The drawing under review shows one solid part. Ordinate dimensions are in mm from its lowest x, y, z. A direction names the side the tool comes from. Coordinates: 2 decimals unless noted, no trailing zeros. Loops run counter-clockwise (first coordinate to the right, second up) from the corner with the lowest first, then second, coordinate; pieces in that order, holes last.
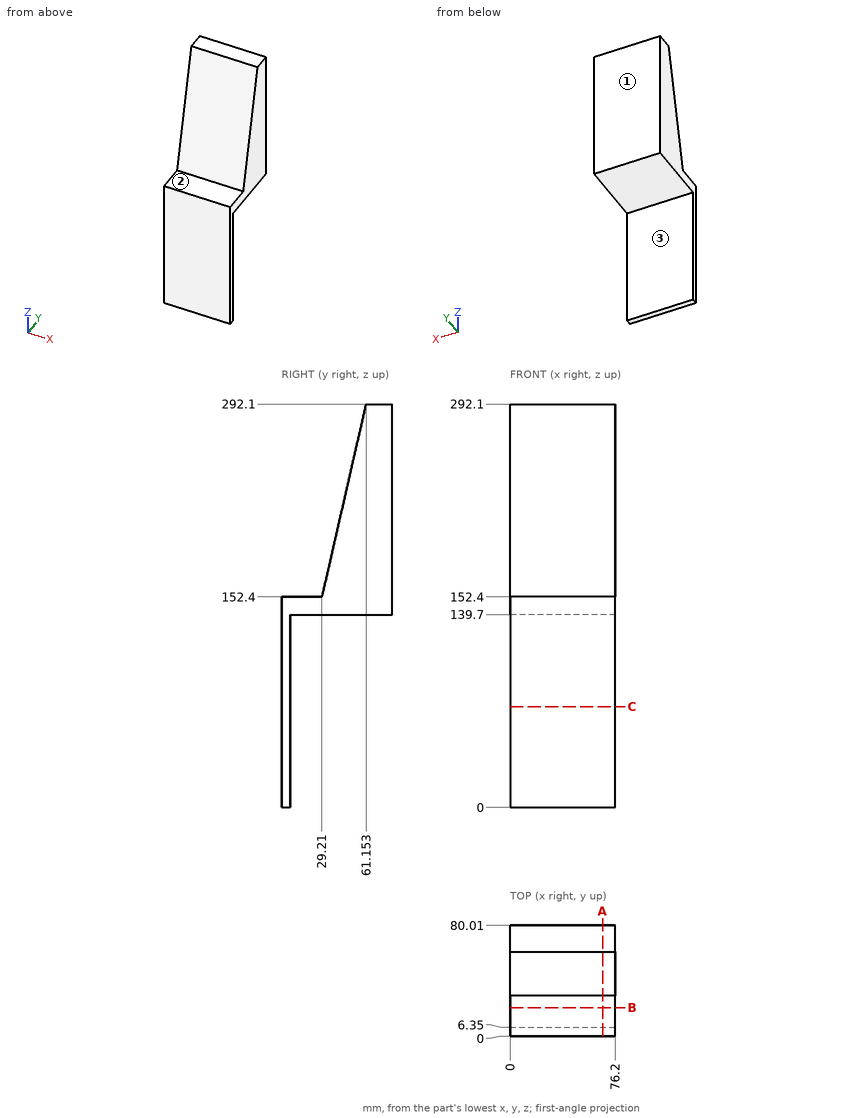
Q1. Take a section at C-C, the plane z = 73. Write out the cut boundary in (x, y).
Q2. Take a section at B-B, the plane y = 20.5. Write out the cut boundary in (x, z).
Q3. Take a section at A-A, the plane x = 67. Write out the cut boundary in (y, z).
Q4. For line 1 (Y direction, x = 44, z = 18); line 2 (Z direction, x = 73, y = 22); line 3 (Z direction, x = 61, y = 64.5), list the stretches that pass through material, from the lowest coordinate up.
Q5. Machinability: for the marked faces 1, 2 and 3, which of the approach directions +Z, -Z, +X, -X, +Y, -Y give a long, thin tool a straight path to every point of the face, cutting with its end or side? Answer none if there is none.
Q6. Clearance check with flat-ended pins moving along their axes: pin 1 Ø8 at (x, z) = (25.5, 99) entering from +Y; pin 2 Ø1 at (x, y) = (44, 14) entering from +Z; pin 3 Ø22 at (x, y) = (24, 56) entering from -Z. State where each tip first meets the part, or that it passes through.
Entries:
1. outline: (0, 0) - (76.2, 0) - (76.2, 6.35) - (0, 6.35) - close
2. outline: (0, 139.7) - (76.2, 139.7) - (76.2, 152.4) - (0, 152.4) - close
3. outline: (0, 0) - (6.35, 0) - (6.35, 139.7) - (80.01, 139.7) - (80.01, 292.1) - (61.15, 292.1) - (29.21, 152.4) - (0, 152.4) - close
4. line 1: y = 0 to 6.35
4. line 2: z = 139.7 to 152.4
4. line 3: z = 139.7 to 292.1
5. face 1: +Z, -Z, +X, -X, +Y
5. face 2: +Z, +X, -X, -Y
5. face 3: -Z, +X, -X, +Y
6. pin 1: stops at y = 6.35
6. pin 2: stops at z = 152.4
6. pin 3: stops at z = 139.7
